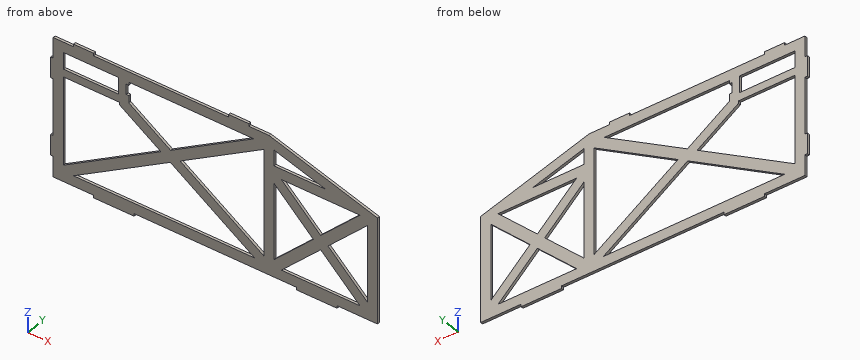
from build123d import *

# Parameters (mm, degrees)
SKETCH1_W           = 69.596
SKETCH1_H           = 20.4724
BOSS_EXTRUDE1_DEPTH = 3.175


with BuildPart() as part:
    # Sketch1 → Boss-Extrude1 (new body)
    with BuildSketch(Plane(origin=(0, 0, 0), x_dir=(1, 0, 0), z_dir=(0, 1, 0))):
        Polygon((135.5725, -85.725), (271.8181, -44.704), (271.8181, 85.725), (221.0181, 85.725), (221.0181, 88.9), (170.2181, 88.9), (170.2181, 85.725), (135.5725, 85.725), (-33.9725, 85.725), (-33.9725, 88.9), (-84.7725, 88.9), (-84.7725, 85.725), (-135.5725, 85.725), (-135.5725, 60.325), (-138.7475, 60.325), (-138.7475, 34.925), (-135.5725, 34.925), (-135.5725, -34.925), (-138.7475, -34.925), (-138.7475, -60.325), (-135.5725, -60.325), (-135.5725, -85.725), (-110.1725, -85.725), (-110.1725, -88.9), (-84.7725, -88.9), (-84.7725, -85.725), (84.7725, -85.725), (84.7725, -88.9), (110.1725, -88.9), (110.1725, -85.725), align=None)
        Polygon((191.30257064, 17.3355), (141.9225, -29.593760892), (141.9225, 64.264760892), align=None, mode=Mode.SUBTRACT)
        Polygon((209.73802936, 17.3355), (259.1181, -29.593760892), (259.1181, 64.264760892), align=None, mode=Mode.SUBTRACT)
        Polygon((141.9225, -51.054), (141.9225, -70.549992123), (206.675751855, -51.054), align=None, mode=Mode.SUBTRACT)
        Polygon((-40.5765, -56.4388), (-40.5765, -47.477682668), (12.060198108, -12.486286049), (116.555282623, -73.025), (-40.5765, -73.025), (-40.5765, -69.1388), (-43.7515, -69.1388), (-43.7515, -56.4388), align=None, mode=Mode.SUBTRACT)
        Polygon((-110.205282623, 73.025), (117.75227551, 73.025), (11.599803294, 2.457821761), align=None, mode=Mode.SUBTRACT)
        Polygon((-122.8725, 65.686309832), (-122.8725, -43.0276), (-52.04672449, -43.0276), (-52.04672449, -39.8526), (-0.197624716, -5.384776605), align=None, mode=Mode.SUBTRACT)
        with Locations((-88.0745, -62.7888)):
            Rectangle(SKETCH1_W, SKETCH1_H, mode=Mode.SUBTRACT)
        Polygon((129.2225, 65.399917332), (129.2225, -65.686309832), (23.857626118, -4.643687684), align=None, mode=Mode.SUBTRACT)
        Polygon((151.14022936, 73.025), (249.90037064, 73.025), (200.5203, 26.095739108), align=None, mode=Mode.SUBTRACT)
        Polygon((151.14022936, -38.354), (249.90037064, -38.354), (200.5203, 8.575260892), align=None, mode=Mode.SUBTRACT)
    extrude(amount=BOSS_EXTRUDE1_DEPTH)


solid = part.part
Can you work these out from the model? Positions are in its coordinate system, mm. Give positions to 0.01 mm unless a question says otherwise; leave off trailing zeros. Loops run counter-clockwise (first coordinate to the right, second up) from the corner with the lowest first, then second, coordinate; pieces in that order, holes last. Notation, with made-up numbers: (40, -20.75) -> (85, -20.75) arc R18 cw to (85, -6.75) -> close; hole circle Ø3 at (-34, 10). An arc over 180 degrees is marked (long way). Write item = value, one per line.
1) Suppose I cut it at C-C on y = 1.8. Give the number of separate pieces and of enclosed holes in the cut face, then the cut area to 3 significant figures.
Check result:
separate_pieces = 1
enclosed_holes = 10
area = 28,000 mm2
2) Suppose I cut it at B-B on x = 157.5. Write out the boundary of the cut face in (y, z) (3 decimals).
Check result:
outline = (0, -85.725) -> (3.175, -85.725) -> (3.175, -73.025) -> (0, -73.025) -> close; (0, -66.981) -> (3.175, -66.981) -> (3.175, -49.46) -> (0, -49.46) -> close; (0, 14.789) -> (3.175, 14.789) -> (3.175, 32.31) -> (0, 32.31) -> close; (0, 38.354) -> (3.175, 38.354) -> (3.175, 51.054) -> (0, 51.054) -> close; (0, 65.86) -> (3.175, 65.86) -> (3.175, 79.123) -> (0, 79.123) -> close
3) Will these pins go through, and if not, where does the flat tip stop? pin 1 (1.6 mm diameter, centred on x = 177.5, y = 2.5, fed in from +Z); pin 2 (1 mm diameter, centred on x = -57, z = 54, fed in from -Y); pin 3 (1 mm diameter, centred on x = -9.5, y = 1, fed in from +Z) (3 decimals); pin 4 (1 mm diameter, centred on y = 2, z = -20, fed in from -X).
Check result:
pin_1 = 73.34
pin_2 = through
pin_3 = 85.725
pin_4 = -135.57
4) Suppose I cut it at A-A on z = -44. Write out the boundary of the cut face in (x, y) (1 decimal), then the cut area to 3 significant figures.
Check result:
outline = (-138.7, 0) -> (-122.9, 0) -> (-122.9, 3.2) -> (-138.7, 3.2) -> close; (-85.4, 0) -> (-60.1, 0) -> (-60.1, 3.2) -> (-85.4, 3.2) -> close; (74.1, 0) -> (97, 0) -> (97, 3.2) -> (74.1, 3.2) -> close; (129.2, 0) -> (141.9, 0) -> (141.9, 3.2) -> (129.2, 3.2) -> close; (163.2, 0) -> (181.7, 0) -> (181.7, 3.2) -> (163.2, 3.2) -> close; (219.4, 0) -> (237.8, 0) -> (237.8, 3.2) -> (219.4, 3.2) -> close; (259.1, 0) -> (271.8, 0) -> (271.8, 3.2) -> (259.1, 3.2) -> close
area = 401 mm2
5) Suppose I cut it at D-D on x = -106. Write out the boundary of the cut face in (y, z) (3 decimals).
Check result:
outline = (0, -85.725) -> (3.175, -85.725) -> (3.175, -73.025) -> (0, -73.025) -> close; (0, -70.589) -> (3.175, -70.589) -> (3.175, -55.911) -> (0, -55.911) -> close; (0, 43.028) -> (3.175, 43.028) -> (3.175, 52.553) -> (0, 52.553) -> close; (0, 73.025) -> (3.175, 73.025) -> (3.175, 88.9) -> (0, 88.9) -> close
6) I need wall thicknesses on L1, parallel to X at y = 2.6, z = 39; L2, parallel to Z at x = 239, y = 1.75 (3 decimals); L3, parallel to Z at x = 220, y = 0.3 (3 decimals). Which ranges of each line are inside material? Lowest first, please. Write a range as from..to.
Check result:
L1 = -138.75..-122.87, -50.76..-27.82, 57.83..83.16, 129.22..271.82
L2 = -85.725..-73.025, -62.666..-45.145, 10.474..27.995, 38.354..54.585
L3 = -88.9..-73.025, -44.609..-27.088, -7.583..9.938, 38.354..60.305
